Geometry check sheet. Reference: the model listing, model coordinates, mm. Round coordinates to 2 decimals unless told otherwise and drop trailing zeros. Order: outer loops, then holes, each group sorted by start corner. A loop starts at its lowest first (then second) coordinate and runs counter-clockwise, first axis right, second up.
(1) Go/stop test with a flat-tipped pin: pin 1 (2 mm diameter, centred on y = -1, z = -1.5, fed in from +X). Record where the tip stops, or that it passes through.
(2) Sectioned sample at B-B (z = -5.25). Record the boundary of the cut face in (x, y) (3 decimals).
(3) Release check for a two-part mould opening along Z. For faces 1 (the face through (-15, 0, -6.35)), 2 (the face through (-15, -3.175, -3)), 3 (the face through (-24.04, 0.63, -1.65)) record: +Z half, -Z half, draft (parallel to the pull), parting line (faces both ways), or undercut.
(4) Sectioned sample at C-C (x = -25.5). Record the boundary of the cut face in (y, z) (3 decimals).
(5) Sectioned sample at A-A (x = -12.7). Record the boundary of the cut face in (y, z) (3 decimals).
(6) Material ranges on line 1 along X through (y, z) = (0, -5); line 2 along Y through (x, z) = (-12.7, -2.75) (3 decimals), recorded low to high.
(7) Sectioned sample at D-D (y = -0.5). Give the number of separate pieces and of enclosed holes in the cut face, plus the area to 3 significant figures.
Autodesk Inventor part; units mm, degrees
ref_plane "YZ Plane" through (0, 0, 0) normal (1, 0, 0) x (0, 1, 0)
ref_plane "XZ Plane" through (0, 0, 0) normal (0, 1, 0) x (-1, 0, 0)
ref_plane "XY Plane" through (0, 0, 0) normal (0, 0, 1) x (1, 0, 0)
sketch "Sketch1" plane through (0, 0, 0) normal (0, 0, 1) x (1, 0, 0)
  line L0 (0, 4.445) -> (0, -4.445)
  line L1 (-38.1, 0) -> (6.35, 0)
  line L2 (-30.48, -3.175) -> (0, -3.175)
  line L3 (0, -3.175) -> (0, 3.175)
  line L4 (0, 3.175) -> (-30.48, 3.175)
  line L5 (-30.48, 3.175) -> (-30.48, -3.175)
  line L6 (-30.48, -3.175) -> (0, 3.175) construction
  line L7 (0, -3.175) -> (-30.48, 3.175) construction
  point P0 (0, 0)
  point P1 (-15.24, 0)
  point P2 (-6.35, 0)
  point P3 (-12.7, 0)
  point P4 (-19.05, 0)
  point P5 (-25.4, 0)
  point P6 (-31.75, 0)
  dimension "d0" = 6.35
  dimension "d1" = 30.48
  dimension "d2" = 6.35
  dimension "d3" = 6.35
  dimension "d4" = 6.35
  dimension "d5" = 6.35
  dimension "d6" = 6.35
extrude "Extrusion1" add sketch "Sketch1" against normal blind 6.35
hole "Hole1" at (-6.35, 0, 0) at (-12.7, 0, 0) direction (0, 0, -1) diameter 2.6416 end through all
hole "Hole2" [suppressed]
fillet "Fillet1" [suppressed]
sketch "Sketch2" plane through (-30.48, -3.175, 0) normal (-1, 0, 0) x (0, 0, 1)
  line L0 (0, 6.35) -> (0, 0)
  line L1 (0, 6.35) -> (-6.35, 6.35)
  line L2 (-6.35, 0) -> (-6.35, 6.35)
  line L3 (0, 0) -> (-6.35, 0)
  line L4 (-6.35, 0) -> (-6.35, 6.35) construction
  line L5 (-6.35, 6.35) -> (0, 0) construction
  point P0 (0, 3.175)
  point P1 (-3.175, 3.175)
hole "Hole3" at (-30.48, 0, -3.175) direction (1, 0, 0) diameter 3.302 depth 12.7 tip angle 118
properties part number "J010309" material "ALUMINUM, 6061-T651"
Answer below:
1. pin 1: stops at x = 0
2. outline: (-30.48, -3.175) - (0, -3.175) - (0, 3.175) - (-30.48, 3.175) - close; hole circle Ø2.642 at (-12.7, 0); hole circle Ø2.642 at (-6.35, 0)
3. face 1: -Z half
3. face 2: draft
3. face 3: undercut
4. outline: (-3.175, -6.35) - (3.175, -6.35) - (3.175, 0) - (-3.175, 0) - close; hole circle Ø3.302 at (0, -3.175)
5. outline: (-3.175, -6.35) - (-1.321, -6.35) - (-1.321, 0) - (-3.175, 0) - close; (1.321, -6.35) - (3.175, -6.35) - (3.175, 0) - (1.321, 0) - close
6. line 1: x = -30.48 to -14.02, -11.38 to -7.67, -5.03 to 0
6. line 2: y = -3.175 to -1.321, 1.321 to 3.175
7. separate pieces: 3
7. enclosed holes: 0
7. area: 121 mm2
